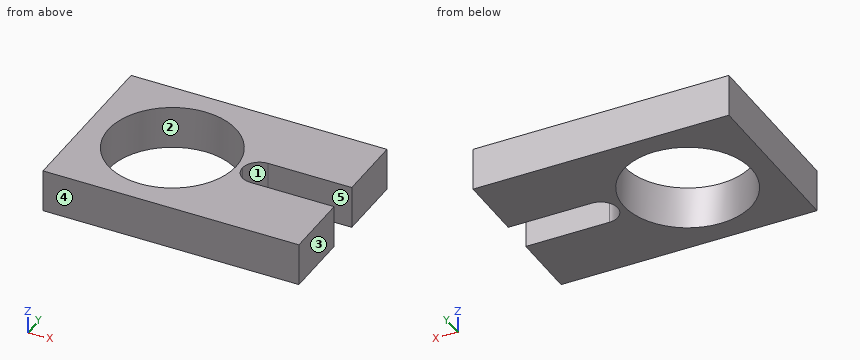
```python
from build123d import *

# Parameters (mm, degrees)
F0_R     = 3.75
F1_DEPTH = 2.5
F2_R     = 1
F3_R     = 0.99999


# Not quite as in the source:
# - a fillet or chamfer is up to 0.001 mm smaller than in the source, because OpenCascade refuses the exact size


with BuildPart() as f1:
    # F0 (on Top) → F1 (new body)
    with BuildSketch(Plane.XY):
        Polygon((10, 5), (-5, 5), (-5, -5), (10, -5), (10, -2.5), (10, -1), (4.1, -1), (4.1, 1), (10, 1), (10, 2.5), align=None)
        Circle(F0_R, mode=Mode.SUBTRACT)
    extrude(amount=F1_DEPTH)

    # F2
    f2_edges = [f1.edges().sort_by_distance(p)[0] for p in [
        (4.1, 1, 1.25),
    ]]
    fillet(f2_edges, radius=F2_R)

    # F3 (radius 1 in the source; OpenCascade refuses exactly that, so slightly less here)
    f3_edges = [f1.edges().sort_by_distance(p)[0] for p in [
        (4.1, -1, 1.25),
    ]]
    fillet(f3_edges, radius=F3_R)


solid = f1.part
```
The model under review builds one solid part; all positions refer to its coordinate system, in mm. Face numbers are marked on the shaded views. A direction names the side the tool comes from. Coordinates: 2 decimals unless noted, no trailing zeros. Write each loop counter-clockwise with the first axis right and the second up, starting at its lowest first coordinate (ties: lowest second). Pieces come first, ordered by that corner, then holes. Notation, with made-up numbers: (-25, -7) -> (-6, -7) arc R21 cw to (-6, 5) -> close; hole circle Ø4 at (-29, 61). An arc over 180 degrees is marked (long way). One line per item, written item: value. Start each with the question number.
Q1. Add section B-B, the plane x = 7.25. Give the boundary of the cut face in (y, z), then the cut area to 3 significant figures.
Q2. For the marked faces 1 and 2, list the 3-axis set-ups (+Z, -Z, +X, -X, +Y, -Y) from which the entire face can be reached by the end or side of a thin tool; tool diameter is ignored.
Q3. Add section A-A, the plane y = 2.25. Give the boundary of the cut face in (x, z).
Q4. Clearance check with flat-ended pins moving along their axes: P1, Ø4, axis at x = 3, y = 1, coming from the -Z side; P2, Ø1.5, axis at x = 5.5, y = 0, coming from the +Z side. State where each tip first meets the part, or that it passes through.
Q5. To check wall thickness, follow probe 1 along Y at (x, z) = (0, 1.75); probe 2 along Y at (x, z) = (9.5, 1.8); probe 3 along X at (y, z) = (2, 0.95). State the ranges of each line that lie inside material, in increasing order.
Q6. The part is to be moulded in two halves that separate along Y. For the marked faces 3, 4 and 5, say which applies: +Y half, -Y half, draft (parallel to the pull), parting line (faces both ways), or undercut.
Response:
1. outline: (-5, 0) -> (-1, 0) -> (-1, 2.5) -> (-5, 2.5) -> close; (1, 0) -> (5, 0) -> (5, 2.5) -> (1, 2.5) -> close
1. area: 20.0 mm²
2. face 1: +Z, -Z, +X
2. face 2: +Z, -Z
3. outline: (-5, 0) -> (-3, 0) -> (-3, 2.5) -> (-5, 2.5) -> close; (3, 0) -> (10, 0) -> (10, 2.5) -> (3, 2.5) -> close
4. P1: z = 0
4. P2: through
5. probe 1: -5 to -3.75, 3.75 to 5
5. probe 2: -5 to -1, 1 to 5
5. probe 3: -5 to -3.17, 3.17 to 10
6. face 3: draft
6. face 4: -Y half
6. face 5: undercut
